```python
from build123d import *

# Parameters (mm, degrees)
F0_R     = 20
F0_R_2   = 14.5
F1_DEPTH = 4
F2_R     = 2.5
F3_R     = 17
F4_DEPTH = 1.3


with BuildPart() as f1:
    # F0 (on Top) → F1 (new body)
    with BuildSketch(Plane.XY):
        Circle(F0_R)
        Circle(F0_R_2, mode=Mode.SUBTRACT)
    extrude(amount=F1_DEPTH)

    # F2
    f2_edges = [f1.edges().sort_by_distance(p)[0] for p in [
        (-14.5, 0, 4),
        (-20, 0, 4),
    ]]
    fillet(f2_edges, radius=F2_R)

    # F3 (on Top) → F4 (cut)
    with BuildSketch(Plane.XY):
        Circle(F3_R)
    extrude(amount=F4_DEPTH, mode=Mode.SUBTRACT)


solid = f1.part
```
Geometry check sheet. Reference: the model listing, model coordinates, mm. A direction names the side the tool comes from. Give positions to 0.01 mm unless a question says otherwise; leave off trailing zeros. Loops run counter-clockwise (first coordinate to the right, second up) from the corner with the lowest first, then second, coordinate; pieces in that order, holes last. Notation, with made-up numbers: M -3,-19 L 1,-19 A12 cw 1,4 Z; hole C 86,-38.5 d2. An arc over 180 degrees is marked long. Write item = value, one per line. Start each with the question number.
1. Tool access check on faces 1 (the face through (13, 8, 1.3)), 2 (the face through (-3, 17, 4)). Record the directions out of +Z, -Z, +X, -X, +Y, -Y that give a thin tool (end or side, any length) a straight path to the whole face; none if there is none.
2. Section check A-A, the plane x = 0. Enter the section's corners in (y, z), plus the area to 3 significant figures.
3. Section check C-C, the plane z = 0.7. Enter the section's corners in (x, y), plus the area to 3 significant figures.
4. Draft check along Y on faces 3 (the face through (-9, -15, 0)), 4 (the face through (-4.336, -19.524, 0.74)), 5 (the face through (9.139, 14.334, 0.641)). Enter one of: +Y half, -Y half, draft (parallel to the pull), parting line (faces both ways), or undercut.
5. Thickness scan on probe 1 along Y at (x, z) = (0, 0.5); probe 2 along Y at (x, z) = (0, 1.4); probe 3 along X at (y, z) = (-2.5, 1.6). Record the ranges inside material, lowest first.
6. Go/stop test with flat-tipped pins: P1, Ø2, axis at x = 3.5, z = 3, coming from the +Y side; P2, Ø2, axis at x = 16, y = 4, coming from the +Z side; P3, Ø2, axis at x = 14, y = -14.5, coming from the +Z side. Record where each tip stops, or that it passes through.
Values follow:
q1.face_1 = -Z
q1.face_2 = +Z, +X, -X, +Y, -Y
q2.outline = M -20,0 L -17,0 L -17,1.3 L -14.5,1.3 L -14.5,1.5 A2.5 ccw -17,4 L -17.5,4 A2.5 ccw -20,1.5 Z; M 14.5,1.3 L 17,1.3 L 17,0 L 20,0 L 20,1.5 A2.5 ccw 17.5,4 L 17,4 A2.5 ccw 14.5,1.5 Z
q2.area = 32.1 mm^2
q3.outline = C 0,0 d40; hole C 0,0 d34
q3.area = 349 mm^2
q4.face_3 = draft
q4.face_4 = parting line
q4.face_5 = undercut
q5.probe_1 = -20 to -17, 17 to 20
q5.probe_2 = -20 to -14.5, 14.5 to 20
q5.probe_3 = -19.84 to -14.28, 14.28 to 19.84
q6.P1 = 19.69
q6.P2 = 4
q6.P3 = 3.37
